Autodesk Inventor part; units mm, degrees
ref_plane "YZ Plane" through (0, 0, 0) normal (1, 0, 0) x (0, 1, 0)
ref_plane "XZ Plane" through (0, 0, 0) normal (0, 1, 0) x (-1, 0, 0)
ref_plane "XY Plane" through (0, 0, 0) normal (0, 0, 1) x (1, 0, 0)
sketch "Sketch2" plane through (0, 0, 0) normal (1, 0, 0) x (0, 1, 0)
  line L0 (-894.1313, -718.7686) -> (883.8687, -1531.5686)
  line L1 (-894.1313, -667.9686) -> (883.8687, -1480.7686)
  line L2 (-894.1313, -667.9686) -> (883.8687, -667.9686)
  line L3 (-894.1313, -718.7686) -> (-894.1313, -667.9686)
  line L4 (883.8687, -1480.7686) -> (883.8687, -1531.5686)
  point P0 (0, 0)
  dimension "d4" = 1778
  dimension "d5" = 50.8
  dimension "d6" = 50.8
  dimension "d7" = 812.8
extrude "Extrusion2" add sketch "Sketch2" along normal blind 1143
sketch "Sketch3" plane through (0, -894.1313, -667.9686) normal (0, 0.4157598, 0.9094745) x (1, 0, 0)
  line L0 (50.8, 1904.1752) -> (1092.2, 1904.1752)
  line L1 (1092.2, 1904.1752) -> (1092.2, 50.8)
  line L2 (1092.2, 50.8) -> (50.8, 50.8)
  line L3 (50.8, 50.8) -> (50.8, 1904.1752)
  line L4 (0, 0) -> (1143, 0)
  line L5 (1143, 1954.9752) -> (1143, 0)
  line L6 (0, 1954.9752) -> (0, 0)
  line L7 (0, 1954.9752) -> (1143, 1954.9752)
  point P0 (0, 535.4751)
  dimension "d10" = 50.8
  dimension "d11" = 50.8
  dimension "d12" = 50.8
  dimension "d13" = 50.8
extrude "Extrusion3" cut sketch "Sketch3" against normal blind 12.7 contours L0 L1 L2 L3
equation "\"BendRadius\" = Thickness"
equation "\"BendReliefWidth\" = Thickness"
equation "\"BendReliefDepth\" = 0.5 * Thickness"
equation "\"CornerReliefSize\" = 4 * Thickness"
equation "\"MinimumRemnant\" = 2 * Thickness"
equation "\"TransitionRadius\" = BendRadius"
equation "\"JacobiRadiusSize\" = BendRadius"
equation "\"GapSize\" = Thickness"
properties part number "screen"
Input: part model. Units: mm. Frame: model coordinates. Coordinates: 2 decimals unless noted, no trailing zeros. Loops run counter-clockwise (first coordinate to the right, second up) from the corner with the lowest first, then second, coordinate; pieces in that order, holes last. Notation, with made-up numbers: (-33.75, 2) -> (-20.75, 2) arc R26 ccw to (-20.75, 23) -> close; hole circle Ø7 at (72, 38.25). An arc over 180 degrees is marked (long way). One line per item, written item: value.
(1) Pin query (flat end, axial travel): pin 1 Ø2 at (x, y) = (637.5, 235) entering from -Z; pin 2 Ø5 at (x, y) = (323.5, -456.5) entering from +Z; pin 3 Ø2 at (x, y) = (751.5, -25) entering from -Z. Return the tip coordinate at first contact, or that it passes through.
Answer below:
pin 1: stops at z = -1235.4
pin 2: stops at z = -880.85
pin 3: stops at z = -1116.54
(2) Cut plane A-A (x = 998.5). Output: boundary loops of the cut face in (y, z), then the cut area to 3 significant figures.
Answer below:
outline: (-894.13, -718.77) -> (883.87, -1531.57) -> (883.87, -1480.77) -> (837.67, -1459.65) -> (832.39, -1471.2) -> (-853.21, -700.64) -> (-847.93, -689.09) -> (-894.13, -667.97) -> close
area: 66,800 mm2
(3) Draft query along X for faces 1 (the face through (1092.2, 4, -1085)), 2 (the face through (1143, -9, -1098)), 3 (the face through (564.21, 1.387, -1091.315)), 4 (the face through (563, -894.131, -694)). Return one class per face: pulls with the +X half, pulls with the -X half, needs draft (parallel to the pull), parting line crosses it, or undercut.
Answer below:
face 1: undercut
face 2: pulls with the +X half
face 3: undercut
face 4: needs draft
(4) Ray query, line 1 along Z through (x, y) = (1046, 813.5); line 2 along Y through (x, z) = (874, -1113); line 3 along Z through (x, y) = (700, 508). Return the intervals inside material, ascending.
Answer below:
line 1: z = -1499.4 to -1462.57
line 2: y = -31.75 to 48.82
line 3: z = -1359.74 to -1322.91
(5) Cut plane B-B (z = -788.5). Output: boundary loops of the cut face in (x, y).
Answer below:
outline: (0, -741.59) -> (1143, -741.59) -> (1143, -630.47) -> (1092.2, -630.47) -> (1092.2, -661.02) -> (50.8, -661.02) -> (50.8, -630.47) -> (0, -630.47) -> close
